Here's how the part is built. I have some questions about the finished solid (model axes, mm). Face numbers are marked on the shaded views. A direction names the side the tool comes from. Round coordinates to 2 decimals unless told otherwise and drop trailing zeros. Write each loop counter-clockwise with the first axis right and the second up, starting at its lowest first coordinate (ties: lowest second). Pieces come first, ordered by that corner, then holes. Notation, with made-up numbers: M 11,-13 L 35,-13 A34 cw 35,19 Z; hole C 40,63 d9. An arc over 180 degrees is marked long. Use a Markdown table: item, result. Add a question column.
```python
from build123d import *

# Parameters (mm, degrees)
EXTRUDE_1_DEPTH     = 15
SKETCH_2_R          = 3.1
CUT_EXTRUDE_1_DEPTH = 59.566201857
FILLET_1_R          = 5
SKETCH_3_R          = 1.6
CUT_EXTRUDE_2_DEPTH = 55.534392818
FILLET_3_R          = 2
FILLET_4_R          = 5


with BuildPart() as part:
    # ｽｹｯﾁ1 → ﾎﾞｽ - 押し出し1 (new body)
    with BuildSketch(Plane.XY):
        Polygon((0, 0), (0, -30), (40, -30), (40, 0), (43, 0), (43, -33), (-3, -33), (-3, 0), align=None)
    extrude(amount=EXTRUDE_1_DEPTH)

    # ｽｹｯﾁ2 → ｶｯﾄ - 押し出し1 (cut, through all)
    with BuildSketch(Plane(origin=(43, 0, 0), x_dir=(0, 0, -1), z_dir=(1, 0, 0))):
        with Locations((-7.5, -7)):
            Circle(SKETCH_2_R)
    extrude(amount=-CUT_EXTRUDE_1_DEPTH, mode=Mode.SUBTRACT)

    # ﾌｨﾚｯﾄ1
    fillet_1_edges = [part.edges().sort_by_distance(p)[0] for p in [
        (-1.5, 0, 0),
        (41.5, 0, 15),
        (-1.5, 0, 15),
        (41.5, 0, 0),
    ]]
    fillet(fillet_1_edges, radius=FILLET_1_R)

    # ｽｹｯﾁ3 → ｶｯﾄ - 押し出し2 (cut, through all)
    with BuildSketch(Plane(origin=(0, -30, 0), x_dir=(1, 0, 0), z_dir=(0, 1, 0))):
        with Locations(Location((7.5, -7.5, 0), (0, 0, 270))):
            Circle(SKETCH_3_R)
        with Locations(Location((32.5, -7.5, 0), (0, 0, 270))):
            Circle(SKETCH_3_R)
    extrude(amount=-CUT_EXTRUDE_2_DEPTH, mode=Mode.SUBTRACT)

    # ﾌｨﾚｯﾄ3
    fillet_3_edges = [part.edges().sort_by_distance(p)[0] for p in [
        (0, -30, 7.5),
        (40, -30, 7.5),
    ]]
    fillet(fillet_3_edges, radius=FILLET_3_R)

    # ﾌｨﾚｯﾄ4
    fillet_4_edges = [part.edges().sort_by_distance(p)[0] for p in [
        (43, -33, 7.5),
        (-3, -33, 7.5),
    ]]
    fillet(fillet_4_edges, radius=FILLET_4_R)


solid = part.part
```
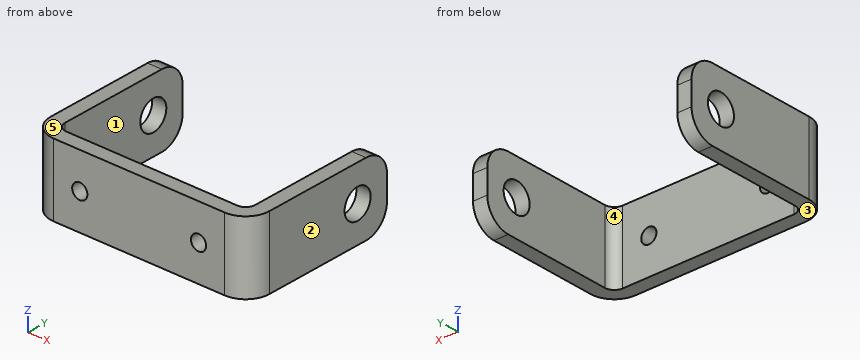
Item 1: Imagine slicing it at B-B on y = -7. List the corners of the cut face in (x, z) for me, plus the area to 3 significant figures.
Item 2: Imagine slicing it at C-C on x = 32.5. List the corners of the cut face in (y, z) for me.
Item 3: For pin 1 Ø3.5 at (x, z) = (7.5, 7.5) entering from +Y, with a flat end and sliding along its axis, tell me the tip position at first contact or that it passes through.
Item 4: Imagine slicing it at A-A on z = 7.5. List the corners of the cut face in (x, y) for me, plus the area to 3 significant figures.
Item 5: Imagine slicing it at D-D on y = -13. List the corners of the cut face in (x, z) for me.
Item 6: On a 3-axis mill with a long thin cutter (end or side, diameter ignored), from which of +Z, -Z, +X, -X, +Y, -Y can I reach the whole of each face in a straight line? I mean the marked faces 4 and 5. Say none if no direction works.
Item 7: If we mould it in two halves opening along X, with no side actions, what happens to the marked faces 1, 2 and 3? For each: +X half, -X half, draft (parallel to the pull), parting line (faces both ways), or undercut.
Item 8: I need wall thicknesses on probe 1 along X at (y, z) = (-11.5, 5.5); probe 2 along Y at (x, z) = (18, 11.5); probe 3 along X at (y, z) = (-30.7, 7.5). Which ranges of each line are inside material? Lowest first, please. Write a range as from..to.
The answers:
| question | item | result |
|---|---|---|
| 1 | outline | M -3,0 L 0,0 L 0,4.4 L -3,4.4 Z; M -3,10.6 L 0,10.6 L 0,15 L -3,15 Z; M 40,0 L 43,0 L 43,4.4 L 40,4.4 Z; M 40,10.6 L 43,10.6 L 43,15 L 40,15 Z |
| 1 | area | 52.8 mm² |
| 2 | outline | M -33,0 L -30,0 L -30,5.9 L -33,5.9 Z; M -33,9.1 L -30,9.1 L -30,15 L -33,15 Z |
| 3 | pin 1 | y = -30 |
| 4 | outline | M -3,-28 A5 ccw 2,-33 L 5.9,-33 L 5.9,-30 L 2,-30 A2 cw 0,-28 L 0,-10.1 L -3,-10.1 Z; M -3,-3.9 L 0,-3.9 L 0,0 L -3,0 Z; M 9.1,-33 L 30.9,-33 L 30.9,-30 L 9.1,-30 Z; M 34.1,-33 L 38,-33 A5 ccw 43,-28 L 43,-10.1 L 40,-10.1 L 40,-28 A2 cw 38,-30 L 34.1,-30 Z; M 40,-3.9 L 43,-3.9 L 43,0 L 40,0 Z |
| 4 | area | 253 mm² |
| 5 | outline | M -3,0 L 0,0 L 0,15 L -3,15 Z; M 40,0 L 43,0 L 43,15 L 40,15 Z |
| 6 | face 4 | +Z, -Z, +Y |
| 6 | face 5 | +Z, +X, -X, +Y, -Y |
| 7 | face 1 | undercut |
| 7 | face 2 | +X half |
| 7 | face 3 | draft |
| 8 | probe 1 | -3..0, 40..43 |
| 8 | probe 2 | -33..-30 |
| 8 | probe 3 | -2.21..5.9, 9.1..30.9, 34.1..42.21 |
